Could you check a few things on this model? Use its own coordinates, in mm. Face numbers are marked on the shaded views. A direction names the side the tool comes from. Round coordinates to 2 decimals unless told otherwise and drop trailing zeros. Loops run counter-clockwise (first coordinate to the right, second up) from the corner with the lowest first, then second, coordinate; pieces in that order, holes last. Notation, with made-up numbers: (86.25, -24.75) - (142.25, -24.75) arc R12 cw to (142.25, -2.75) - close; hole circle Ø11 at (-26.75, -30). An arc over 180 degrees is marked (long way). Use one line per item in the form item = value.
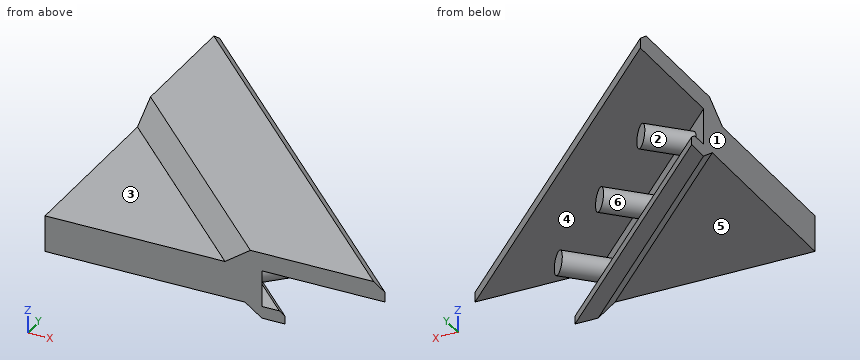
```python
from build123d import *

# Parameters (mm, degrees)
PAD_DEPTH              = 4.55
SKETCH001_R            = 2.9
PAD001_DEPTH           = 12
LINEARPATTERN_COUNT    = 2
LINEARPATTERN_PITCH    = 30
LINEARPATTERN001_COUNT = 2
LINEARPATTERN001_PITCH = 30
PAD002_DEPTH           = 4.5
CHAMFER_SIZE           = 4.49
CHAMFER001_SIZE        = 2
PAD003_DEPTH           = 3
CHAMFER002_SIZE        = 2.99
CHAMFER003_SIZE        = 1


with BuildPart() as part:
    # Sketch → Pad (new body, symmetric)
    with BuildSketch(Plane.XY):
        Polygon((0, 0), (54.2, 0), (0, 54.2), align=None)
    extrude(amount=PAD_DEPTH, both=True)

    # Sketch001 (on Face2 of Pad) → Pad001 (join)
    with BuildSketch(Plane(origin=(27.1, 27.1, 0), x_dir=(-0.707107, 0.707107, 0), z_dir=(0.707107, 0.707107, 0))):
        Circle(SKETCH001_R)
    pad001 = extrude(amount=PAD001_DEPTH)

    # LinearPattern: Pad001 ×2
    with Locations(*[Vector(-0.707107, 0.707107, 0) * (i * LINEARPATTERN_PITCH) for i in range(1, LINEARPATTERN_COUNT)]):
        add(pad001)

    # LinearPattern001: Pad001 ×2
    with Locations(*[Vector(0.707107, -0.707107, 0) * (i * LINEARPATTERN001_PITCH) for i in range(1, LINEARPATTERN001_COUNT)]):
        add(pad001)

    # Sketch002 (on Face5 of LinearPattern001) → Pad002 (join)
    with BuildSketch(Plane.XY.offset(4.55)):
        Polygon((0, 85), (0, 45), (45, 0), (85, 0), align=None)
    extrude(amount=PAD002_DEPTH)

    # Chamfer
    chamfer_edges = [part.edges().sort_by_distance(p)[0] for p in [
        (22.5, 22.5, 9.05),
    ]]
    chamfer(chamfer_edges, length=CHAMFER_SIZE)

    # Chamfer001
    chamfer001_edges = [part.edges().sort_by_distance(p)[0] for p in [
        (42.5, 42.5, 9.05),
    ]]
    chamfer(chamfer001_edges, length=CHAMFER001_SIZE)

    # Sketch003 (on Face11 of Chamfer001) → Pad003 (join)
    with BuildSketch(Plane(origin=(0, 0, -4.55), x_dir=(1, 0, 0), z_dir=(0, 0, -1))):
        Polygon((60, 0), (50, 0), (0, -50), (0, -60), align=None)
    extrude(amount=PAD003_DEPTH)

    # Chamfer002
    chamfer002_edges = [part.edges().sort_by_distance(p)[0] for p in [
        (25, 25, -7.55),
    ]]
    chamfer(chamfer002_edges, length=CHAMFER002_SIZE)

    # Chamfer003
    chamfer003_edges = [part.edges().sort_by_distance(p)[0] for p in [
        (30, 30, -4.55),
    ]]
    chamfer(chamfer003_edges, length=CHAMFER003_SIZE)


solid = part.part
```
1. We'd pull the mould along X, two halves only. Please class the marked faces 1, 2 and 3: +X half, -X half, draft (parallel to the pull), parting line (faces both ways), or undercut.
Solution:
face_1 = -X half
face_2 = undercut
face_3 = draft
2. If we section it at C-C, the plane x = 71.5: Write out the boundary of the cut face in (y, z), plus the area to 3 significant figures.
Solution:
outline = (0, 4.55) - (13.5, 4.55) - (13.5, 7.05) - (10.67, 9.05) - (0, 9.05) - close
area = 57.9 mm^2
3. On a 3-axis mill with a long thin cutter (end or side, diameter ignored), from which of +Z, -Z, +X, -X, +Y, -Y can I reach the whole of each face in a straight line? I mean the marked faces 4, 5 and 6. Say none if no direction works.
Solution:
face_4 = +X, +Y
face_5 = -Z, -X, -Y
face_6 = none
4. Please list where these lines run through material, in increasing order: line 1 along Z through (x, y) = (75, 4.5); line 2 along X through (y, z) = (9.5, 0.5); line 3 along Z through (x, y) = (20.5, 9).
Solution:
line_1 = 4.55 to 9.05
line_2 = 0 to 44.7, 47.89 to 55.97
line_3 = -4.55 to 4.55
5. For P1, Ø3, axis at y = 61.5, z = 7, coming from the +X side; P2, Ø10, axis at x = 9, y = 9, coming from the -Z side; P3, Ø5, axis at x = 12, z = 2, coming from the +Y side, each with a flat end and sliding along its axis, tell me the tip position at first contact or that it passes through.
Solution:
P1 = 25
P2 = -4.55
P3 = 58.85
6. If we section it at D-D, the plane x = 56.5: Count the separate pieces of the cut face and the enclosed holes in it, plus the area to 3 significant figures.
Solution:
separate_pieces = 3
enclosed_holes = 0
area = 157 mm^2
7. If we section it at B-B, the plane z = 1.75: Write out the boundary of the cut face in (x, y).
Solution:
outline = (0, 0) - (54.2, 0) - (49.95, 4.25) - (58.43, 12.74) - (55.16, 16.01) - (46.68, 7.52) - (28.74, 25.46) - (37.22, 33.95) - (33.95, 37.22) - (25.46, 28.74) - (7.52, 46.68) - (16.01, 55.16) - (12.74, 58.43) - (4.25, 49.95) - (0, 54.2) - close
